Geometry check sheet. Reference: the model listing, model coordinates, mm. A direction names the side the tool comes from. Round coordinates to 2 decimals unless told otherwise and drop trailing zeros.
(1) Material ranges on line 1 along Y through (x, z) = (-5.25, 316); line 2 along X through (y, z) = (10, 303.5); line 3 along Y through (x, z) = (-10.75, 283.5), recorded low to high.
(2) Release check for a two-part mould opening along X. For faces 3 (the face through (12.7, 17, 323)), 4 (the face through (-12.7, 17, 323)), 5 (the face through (10.16, 15, 323)), 6 (the face through (-11.45, 0.38, 555.01)) record: +X half, -X half, draft (parallel to the pull), parting line (faces both ways), or undercut.
(3) Set-up check for faces 1 (the face through (0, -22.81, 323)), 2 (the face through (11.412, -11.715, 130.208)): record each of +Z, -Z, +X, -X, +Y, -Y from which the full face is reachable in a straight line by a thin tool's end or side.
(4) Go/stop test with a flat-tipped pin: pin 1 (6.5 mm diameter, centred on x = 0, z = 266.7, fed in from +Y). Record where the tip stops, or that it passes through.
from build123d import *

# Parameters (mm, degrees)
CROQUIS1_W              = 25.4
CROQUIS1_H              = 50.7
CROQUIS1_W_2            = 20.32
CROQUIS1_H_2            = 45.62
SALIENTE_EXTRUIR1_DEPTH = 655
CROQUIS2_R              = 2.07
CORTAR_EXTRUIR1_DEPTH   = 658.082019234
CROQUIS3_R              = 14.275
CORTAR_EXTRUIR2_DEPTH   = 700
CROQUIS8_R              = 19.05
CROQUIS8_R_2            = 14.2748
CORTAR_EXTRUIR5_DEPTH   = 700
CROQUIS10_R             = 2.02
CORTAR_EXTRUIR7_DEPTH   = 656.982303496
CROQUIS12_R             = 2.02
CORTAR_EXTRUIR8_DEPTH   = 656.982303496
CROQUIS15_R             = 2.409528967
CROQUIS15_R_2           = 2.413
CORTAR_EXTRUIR10_DEPTH  = 656.982303496


with BuildPart() as part:
    # Croquis1 → Saliente-Extruir1 (new body)
    with BuildSketch(Plane.XY):
        Rectangle(CROQUIS1_W, CROQUIS1_H)
        Rectangle(CROQUIS1_W_2, CROQUIS1_H_2, mode=Mode.SUBTRACT)
    extrude(amount=SALIENTE_EXTRUIR1_DEPTH)

    # Croquis2 → Cortar-Extruir1 (cut, through all)
    with BuildSketch(Plane(origin=(0, 25.35, 0), x_dir=(1, 0, 0), z_dir=(0, 1, 0))):
        with Locations(Location((0, -12.7, 0), (0, 0, 270))):
            Circle(CROQUIS2_R)
        with Locations(Location((0, -38.1, 0), (0, 0, 270))):
            Circle(CROQUIS2_R)
        with Locations(Location((0, -63.5, 0), (0, 0, 270))):
            Circle(CROQUIS2_R)
        with Locations(Location((0, -88.9, 0), (0, 0, 270))):
            Circle(CROQUIS2_R)
        with Locations(Location((0, -114.3, 0), (0, 0, 270))):
            Circle(CROQUIS2_R)
        with Locations(Location((0, -139.7, 0), (0, 0, 270))):
            Circle(CROQUIS2_R)
        with Locations(Location((0, -165.1, 0), (0, 0, 270))):
            Circle(CROQUIS2_R)
        with Locations(Location((0, -190.5, 0), (0, 0, 270))):
            Circle(CROQUIS2_R)
        with Locations(Location((0, -215.9, 0), (0, 0, 270))):
            Circle(CROQUIS2_R)
        with Locations(Location((0, -241.3, 0), (0, 0, 270))):
            Circle(CROQUIS2_R)
        with Locations(Location((0, -266.7, 0), (0, 0, 270))):
            Circle(CROQUIS2_R)
        with Locations(Location((0, -292.1, 0), (0, 0, 270))):
            Circle(CROQUIS2_R)
        with Locations(Location((0, -317.5, 0), (0, 0, 270))):
            Circle(CROQUIS2_R)
        with Locations(Location((0, -342.9, 0), (0, 0, 270))):
            Circle(CROQUIS2_R)
        with Locations(Location((0, -368.3, 0), (0, 0, 270))):
            Circle(CROQUIS2_R)
        with Locations(Location((0, -393.7, 0), (0, 0, 270))):
            Circle(CROQUIS2_R)
        with Locations(Location((0, -419.1, 0), (0, 0, 270))):
            Circle(CROQUIS2_R)
        with Locations(Location((0, -444.5, 0), (0, 0, 270))):
            Circle(CROQUIS2_R)
        with Locations(Location((0, -469.9, 0), (0, 0, 270))):
            Circle(CROQUIS2_R)
        with Locations(Location((0, -495.3, 0), (0, 0, 270))):
            Circle(CROQUIS2_R)
        with Locations(Location((0, -520.7, 0), (0, 0, 270))):
            Circle(CROQUIS2_R)
        with Locations(Location((0, -546.1, 0), (0, 0, 270))):
            Circle(CROQUIS2_R)
        with Locations(Location((0, -571.5, 0), (0, 0, 270))):
            Circle(CROQUIS2_R)
        with Locations(Location((0, -596.9, 0), (0, 0, 270))):
            Circle(CROQUIS2_R)
        with Locations(Location((0, -622.3, 0), (0, 0, 270))):
            Circle(CROQUIS2_R)
        with Locations(Location((0, -647.7, 0), (0, 0, 270))):
            Circle(CROQUIS2_R)
    extrude(amount=-CORTAR_EXTRUIR1_DEPTH, mode=Mode.SUBTRACT)

    # Croquis3 → Cortar-Extruir2 (cut)
    with BuildSketch(Plane.ZY.offset(12.7)):
        with Locations(Location((327.5, 0, 0), (0, 0, 270))):
            Circle(CROQUIS3_R)
    extrude(amount=-CORTAR_EXTRUIR2_DEPTH, mode=Mode.SUBTRACT)

    # Croquis8 → Cortar-Extruir5 (cut)
    with BuildSketch(Plane.ZY.offset(12.7)):
        with Locations(Location((114.145124111, -1.474, 0), (0, 0, 270))):
            Circle(CROQUIS8_R)
        with Locations(Location((540.854875889, -1.474, 0), (0, 0, 270))):
            Circle(CROQUIS8_R_2)
    extrude(amount=-CORTAR_EXTRUIR5_DEPTH, mode=Mode.SUBTRACT)

    # Croquis10 → Cortar-Extruir7 (cut, through all)
    with BuildSketch(Plane(origin=(12.7, 0, 0), x_dir=(0, 0, -1), z_dir=(1, 0, 0))):
        with Locations(Location((-496.854875889, -1.45, 0), (0, 0, 90))):
            Circle(CROQUIS10_R)
    extrude(amount=-CORTAR_EXTRUIR7_DEPTH, mode=Mode.SUBTRACT)

    # Croquis12 → Cortar-Extruir8 (cut, through all)
    with BuildSketch(Plane(origin=(12.7, 0, 0), x_dir=(0, 0, -1), z_dir=(1, 0, 0))):
        with Locations(Location((-283.5, 0, 0), (0, 0, 90))):
            Circle(CROQUIS12_R)
    extrude(amount=-CORTAR_EXTRUIR8_DEPTH, mode=Mode.SUBTRACT)

    # Croquis15 → Cortar-Extruir10 (cut, through all)
    with BuildSketch(Plane.ZY.offset(12.7)):
        with Locations(Location((137.957624111, -1.474, 0), (0, 0, 270))):
            Circle(CROQUIS15_R)
        with Locations(Location((90.332624111, -1.474, 0), (0, 0, 270))):
            Circle(CROQUIS15_R_2)
    extrude(amount=-CORTAR_EXTRUIR10_DEPTH, mode=Mode.SUBTRACT)


solid = part.part
Answer below:
1. line 1: y = -25.35 to -22.81, 22.81 to 25.35
1. line 2: x = -12.7 to -10.16, 10.16 to 12.7
1. line 3: y = -25.35 to -2.02, 2.02 to 25.35
2. face 3: +X half
2. face 4: -X half
2. face 5: undercut
2. face 6: draft
3. face 1: +Z, -Z
3. face 2: +X, -X
4. pin 1: stops at y = 25.35
